Geometry: final body of the model. Coordinates: model frame, mm. Give positions to 0.01 mm unless a question says otherwise; leave off trailing zeros. Write each loop counter-clockwise with the first axis right and the second up, starting at its lowest first coordinate (ties: lowest second). Pieces come first, ordered by that corner, then holes.
Q1. Cut plane A-A on z = -0.9. Return the cut outline in (x, y).
Q2. Pin query (flat end, axial travel): pin 1 (0.8 mm diameter, centred on y = 106, z = -1, fed in from -X); pin 2 (0.8 mm diameter, centred on x = -946, z = -1, fed in from +Y). Return the tip coordinate at first contact, or that it passes through.
Q3. Cut plane C-C on y = 169.5. Return the cut outline in (x, z).
Q4. Cut plane B-B on y = 77.5. Return the cut outline in (x, z).
Q5. Line query: L1, parallel to X at y = 97, z = -1.4; L2, parallel to Y at x = -753, z = -0.75; L3, parallel to X at y = 48.5, z = -0.1. Output: solid intervals per line, ascending.
```python
from build123d import *

# Parameters (mm, degrees)
CROQUIS1_W            = 1652
CROQUIS1_H            = 495.4
BRIDA_BASE1_DEPTH     = 1.5875
CROQUIS21_W           = 370
CROQUIS21_H           = 160
CORTAR_EXTRUIR2_DEPTH = 10
REDONDEO4_R           = 20
REDONDEO5_R           = 50
REDONDEO6_R           = 20


# Sheet-metal steps are written as plain solids
with BuildPart() as part:
    # Croquis1 → Brida base1 (new body)
    with BuildSketch(Plane.XY):
        with Locations((-270.54091127, -44.567814371)):
            Rectangle(CROQUIS1_W, CROQUIS1_H)
    extrude(amount=-BRIDA_BASE1_DEPTH)

    # Croquis21 → Cortar-Extruir2 (cut)
    with BuildSketch(Plane.XY):
        with Locations((-911.54091127, 123.132185629)):
            Rectangle(CROQUIS21_W, CROQUIS21_H)
    extrude(amount=-CORTAR_EXTRUIR2_DEPTH, mode=Mode.SUBTRACT)

    # Redondeo4
    redondeo4_edges = [part.edges().sort_by_distance(p)[0] for p in [
        (-726.54091127, 43.132185629, -0.79375),
    ]]
    fillet(redondeo4_edges, radius=REDONDEO4_R)

    # Redondeo5
    redondeo5_edges = [part.edges().sort_by_distance(p)[0] for p in [
        (-726.54091127, 203.132185629, -0.79375),
    ]]
    fillet(redondeo5_edges, radius=REDONDEO5_R)

    # Redondeo6
    redondeo6_edges = [part.edges().sort_by_distance(p)[0] for p in [
        (-1096.54091127, 43.132185629, -0.79375),
    ]]
    fillet(redondeo6_edges, radius=REDONDEO6_R)


solid = part.part
```
Data:
1. outline: (-1096.54, -292.27) - (555.46, -292.27) - (555.46, 203.13) - (-676.54, 203.13) arc R50 ccw to (-726.54, 153.13) - (-726.54, 63.13) arc R20 cw to (-746.54, 43.13) - (-1076.54, 43.13) arc R20 ccw to (-1096.54, 23.13) - close
2. pin 1: stops at x = -726.54
2. pin 2: stops at y = 43.13
3. outline: (-723.79, -1.59) - (555.46, -1.59) - (555.46, 0) - (-723.79, 0) - close
4. outline: (-726.54, -1.59) - (555.46, -1.59) - (555.46, 0) - (-726.54, 0) - close
5. L1: x = -726.54 to 555.46
5. L2: y = -292.27 to 43.13
5. L3: x = -732.91 to 555.46
